For this review, take the finished solid that the model builds, in its own axes (mm). A direction names the side the tool comes from. Round coordinates to 2 decimals unless told otherwise and drop trailing zeros. Write each loop counter-clockwise with the first axis right and the second up, starting at its lowest first coordinate (ties: lowest second). Pieces come first, ordered by that corner, then holes.
from build123d import *

# Parameters (mm, degrees)
SKETCH2_W           = 76.718161642
SKETCH2_H           = 45.5
BOSS_EXTRUDE1_DEPTH = 5
CUT_EXTRUDE1_DEPTH  = 10


with BuildPart() as part:
    # Sketch2 → Boss-Extrude1 (new body)
    with BuildSketch(Plane(origin=(0, 0, 0), x_dir=(-1, 0, 0), z_dir=(0, 0, -1))):
        with Locations((184.636580821, -32.25)):
            Rectangle(SKETCH2_W, SKETCH2_H)
    extrude(amount=BOSS_EXTRUDE1_DEPTH)

    # Sketch3 → Cut-Extrude1 (cut)
    with BuildSketch(Plane(origin=(0, 0, -5), x_dir=(-1, 0, 0), z_dir=(0, 0, -1))):
        Polygon((155.9375, -55), (155.9375, -51), (154.4875, -51), (154.4875, -48), (155.9375, -48), (155.9375, -42), (159.8375, -42), (159.8375, -48), (161.2875, -48), (161.2875, -51), (159.8375, -51), (159.8375, -55), align=None)
        Polygon((165.9375, -55), (165.9375, -51), (164.4875, -51), (164.4875, -48), (165.9375, -48), (165.9375, -42), (169.8375, -42), (169.8375, -48), (171.2875, -48), (171.2875, -51), (169.8375, -51), (169.8375, -55), align=None)
    extrude(amount=-CUT_EXTRUDE1_DEPTH, mode=Mode.SUBTRACT)


solid = part.part
(1) For faces 1 (the face through (-184, -32, -5)), 2 (the face through (-165, -48, -3)), 3 (the face through (-165.938, -45, -3)), list the 3-axis set-ups (+Z, -Z, +X, -X, +Y, -Y) from which the entire face can be reached by the end or side of a thin tool; tool diameter is ignored.
Geometry check:
face 1: -Z, +X, -X, +Y, -Y
face 2: +Z, -Z
face 3: +Z, -Z, -Y
(2) For pin 1 Ø3 at (x, z) = (-167.5, -2) entering from -Y, flat-tipped, find the tip position at first contact; note if it passes through.
Geometry check:
pin 1: stops at y = -42
(3) Mouldability with a two-part tool opening along X and no side actions: class faces 4 (the face through (-155.938, -53, -3)), 5 (the face through (-196, -55, -2)), 6 (the face through (-222.996, -33, -2)) as pulls with the +X half, pulls with the -X half, needs draft (parallel to the pull), parting line crosses it, or undercut.
Geometry check:
face 4: undercut
face 5: needs draft
face 6: pulls with the -X half
(4) We need section B-B, the plane z = -2.55. Give the boundary of the cut face in (x, y).
Geometry check:
outline: (-223, -55) - (-169.84, -55) - (-169.84, -51) - (-171.29, -51) - (-171.29, -48) - (-169.84, -48) - (-169.84, -42) - (-165.94, -42) - (-165.94, -48) - (-164.49, -48) - (-164.49, -51) - (-165.94, -51) - (-165.94, -55) - (-159.84, -55) - (-159.84, -51) - (-161.29, -51) - (-161.29, -48) - (-159.84, -48) - (-159.84, -42) - (-155.94, -42) - (-155.94, -48) - (-154.49, -48) - (-154.49, -51) - (-155.94, -51) - (-155.94, -55) - (-146.28, -55) - (-146.28, -9.5) - (-223, -9.5) - close
(5) For line 1 along X through (y, z) = (-49, -0.7); line 2 along Y through (x, z) = (-161, -1.8); line 3 along X through (y, z) = (-43.5, -4.45), list the stretches that pass through material, from the lowest coordinate up.
Geometry check:
line 1: x = -223 to -171.29, -164.49 to -161.29, -154.49 to -146.28
line 2: y = -55 to -51, -48 to -9.5
line 3: x = -223 to -169.84, -165.94 to -159.84, -155.94 to -146.28
(6) We need section A-A, the plane y = -47. Give the boundary of the cut face in (x, z), and give its area (3 significant figures).
Geometry check:
outline: (-223, -5) - (-169.84, -5) - (-169.84, 0) - (-223, 0) - close; (-165.94, -5) - (-159.84, -5) - (-159.84, 0) - (-165.94, 0) - close; (-155.94, -5) - (-146.28, -5) - (-146.28, 0) - (-155.94, 0) - close
area: 345 mm2
